Autodesk Inventor part; units mm, degrees
ref_plane "YZ Plane" through (0, 0, 0) normal (1, 0, 0) x (0, 1, 0)
ref_plane "XZ Plane" through (0, 0, 0) normal (0, 1, 0) x (-1, 0, 0)
ref_plane "XY Plane" through (0, 0, 0) normal (0, 0, 1) x (1, 0, 0)
sketch "Sketch1" plane through (0, 0, 0) normal (0, 0, 1) x (1, 0, 0)
  line L0 (0, 0) -> (-8.7, 0)
  line L1 (-8.7, 0) -> (-8.7, 8.7)
  line L2 (-8.7, 8.7) -> (0, 8.7)
  line L3 (0, 8.7) -> (0, 0)
  dimension "d0" = 8.7
  dimension "d1" = 8.7
extrude "Extrusion1" add sketch "Sketch1" along normal blind 3
sketch "Sketch2" plane through (-8.7, 0, 0) normal (-1, 0, 0) x (0, 0, 1)
  line L0 (0, 8.7) -> (0, 0)
  line L1 (0, 0) -> (3, 0)
  line L2 (3, 0) -> (3, 8.7)
  line L3 (3, 8.7) -> (0, 8.7)
  line L4 (0, 8.7) -> (0, 0)
extrude "Extrusion2" add sketch "Sketch2" along normal blind 3
sketch "Sketch3" plane through (0, 0, 3) normal (0, 0, 1) x (1, 0, 0)
  line L0 (0, 8.7) -> (-11.7, 8.7)
  line L1 (0, 0) -> (-11.7, 0)
  line L2 (-11.7, 8.7) -> (-8.7, 8.7)
  line L3 (-8.7, 8.7) -> (-8.7, 0)
  line L4 (-8.7, 0) -> (-11.7, 0)
  line L5 (-11.7, 0) -> (-11.7, 8.7)
  dimension "d6" = 3
extrude "Extrusion3" add sketch "Sketch3" along normal blind 10
sketch "Sketch5" plane through (0, 0, 0) normal (1, 0, 0) x (0, 0, -1)
  line L0 (0, 8.7) -> (-3, 8.7)
  line L1 (0, 0) -> (-3, 0)
  line L2 (-3, 0) -> (-3, 8.7)
  line L3 (-3, 8.7) -> (0, 8.7)
  line L4 (0, 8.7) -> (0, 0)
  dimension "d9" = 3
extrude "Extrusion4" add sketch "Sketch5" along normal blind 3
sketch "Sketch6" plane through (0, 0, 3) normal (0, 0, 1) x (1, 0, 0)
  line L0 (3, 8.7) -> (-11.7, 8.7)
  line L1 (3, 8.7) -> (0, 8.7)
  line L2 (0, 8.7) -> (0, 0)
  line L3 (0, 0) -> (3, 0)
  line L4 (3, 0) -> (3, 8.7)
extrude "Extrusion5" add sketch "Sketch6" along normal blind 25
properties part number "Hook_TestFit"
For this review, take the finished solid that the model builds, in its own axes (mm). A direction names the side the tool comes from. Round coordinates to 2 decimals unless told otherwise and drop trailing zeros. Order: outer loops, then holes, each group sorted by start corner. A loop starts at its lowest first (then second) coordinate and runs counter-clockwise, first axis right, second up. Notation, with made-up numbers: M -38.5,-7 L -6.5,-7 A34 ccw -6.5,27 Z; hole C -11,-10 d4. An arc over 180 degrees is marked long. Use a Markdown table: item, result. Add a question column.
Item 1: Tool access review of faces 5 (the flat face through (-10, 4, 13)), 6 (the flat face through (-8.7, 4, 8)), 7 (the flat face through (3, 4, 14)): name each direction out of +Z, -Z, +X, -X, +Y, -Y from which nothing blocks a thin tool from reaching the whole face with its end or side.
Item 2: Add section A-A, the plane z = 6. Give the boundary of the cut face in (x, y), then the cut area to 3 significant figures.
Item 3: Insertion check: pin 1 (4.5 mm diameter, centred on y = 2.5, z = 21.5, fed in from -X); pin 2 (3 mm diameter, centred on x = -2.5, z = 9.5, fed in from -Y); pin 3 (1.5 mm diameter, centred on x = -9.5, y = 5.5, fed in from +Z); pin 4 (4.5 mm diameter, centred on x = -3.5, y = 5, fed in from +Z). Each pin has a flat end and moves straight along its axis. Give the tip position at first contact, or say it passes through.
Item 4: To check wall thickness, follow line 1 along X through (y, z) = (3.5, 9); line 2 along X through (y, z) = (3.25, 18.5). State the ranges of each line that lie inside material, in increasing order.
Item 5: Add section C-C, the plane x = -10. Give the boundary of the cut face in (y, z).
Item 6: Add section D-D, the plane z = 15.75. Give the boundary of the cut face in (x, y).
Item 7: Add section B-B, the plane y = 6.5. Give the boundary of the cut face in (x, z), then the cut area to 3 significant figures.
Item 8: Mouldability with a two-part tool opening along X and no side actions: class faces 1 (the flat face through (1, 8.7, 11)), 2 (the flat face through (-11.7, 4, 6)), 3 (the flat face through (-4, 4, 3)), 4 (the flat face through (0, 4, 15)) as released by +X, released by -X, zero draft, split by the parting line, or undercut.
Geometry results:
| question | item | result |
|---|---|---|
| 1 | face 5 | +Z, -X, +Y, -Y |
| 1 | face 6 | +Z, +Y, -Y |
| 1 | face 7 | +Z, -Z, +X, +Y, -Y |
| 2 | outline | M -11.7,0 L -8.7,0 L -8.7,8.7 L -11.7,8.7 Z; M 0,0 L 3,0 L 3,8.7 L 0,8.7 Z |
| 2 | area | 52.2 mm² |
| 3 | pin 1 | stops at x = 0 |
| 3 | pin 2 | passes through |
| 3 | pin 3 | stops at z = 13 |
| 3 | pin 4 | stops at z = 3 |
| 4 | line 1 | x = -11.7 to -8.7, 0 to 3 |
| 4 | line 2 | x = 0 to 3 |
| 5 | outline | M 0,0 L 8.7,0 L 8.7,13 L 0,13 Z |
| 6 | outline | M 0,0 L 3,0 L 3,8.7 L 0,8.7 Z |
| 7 | outline | M -11.7,0 L 3,0 L 3,28 L 0,28 L 0,3 L -8.7,3 L -8.7,13 L -11.7,13 Z |
| 7 | area | 149 mm² |
| 8 | face 1 | zero draft |
| 8 | face 2 | released by -X |
| 8 | face 3 | undercut |
| 8 | face 4 | undercut |
